Here's how the part is built. I have some questions about the finished solid (model axes, mm). A direction names the side the tool comes from. Give positions to 0.01 mm unless a question says otherwise; leave off trailing zeros. Write each loop counter-clockwise with the first axis right and the second up, starting at its lowest first coordinate (ties: lowest second). Pieces come first, ordered by that corner, then holes. Notation, with made-up numbers: (82.5, 34) -> (140.5, 34) arc R17 ccw to (140.5, 51) -> close; hole circle Ø9 at (1, 1). An arc over 180 degrees is marked (long way). Use CSV: the item, a comma, the result in double quotes. Start each with the question number.
(1) For pin 1 Ø3.5 at (x, y) = (-10, 0) entering from +Z; pin 2 Ø4 at (x, y) = (4, -3) entering from +Z, each with a flat end and sliding along its axis, tell me the tip position at first contact or that it passes through.
(2) Which directions (+Z, -Z, +X, -X, +Y, -Y) give clear straight access to the entire face, cutting with the end or side of a thin tool? Please do faces 1 (the cylindrical face through (-8.903, 0.345, 2.014)), 2 (the flat face through (-3.5, 0.1, 3)).
(3) Suppose I cut it at A-A on y = 0. List the corners of the cut face in (x, z) for me, plus the area to 3 significant figures.
(4) If we mould it in two halves opening along Y, with no side actions, what happens to faces 3 (the cylindrical face through (1.617, -0.67, 6.084)), 4 (the cylindrical face through (1.78, 7.18, 1.72)), 5 (the cylindrical face through (-1.78, -7.18, 1.72))? For each: pulls with the +Y half, pulls with the -Y half, needs draft (parallel to the pull), parting line crosses it, or undercut.
(5) Suppose I cut it at B-B on z = 10.25. List the corners of the cut face in (x, y) for me, plus the area to 3 significant figures.
(6) I need wall thicknesses on L1, parallel to Y at x = 10, z = 1.8; L2, parallel to Y at x = 0, z = 6.75; L3, parallel to Z at x = 3.5, y = -0.25. Which ranges of each line are inside material? Lowest first, please. Write a range as [from, to].
from build123d import *

# Parameters (mm, degrees)
F1_DEPTH      = 3
F2_T1_DEPTH   = 24.3364797517
F3_T1_DEPTH   = 14.1373136471
F4_R          = 3.25
F5_DEPTH      = 9
F6_R          = 1.75
F7_DEPTH      = 12.001
F8_SIZE       = 0.5
F4_R_2        = 1.15
F9_DEPTH      = 3.001
F10_SIZE      = 1
F11_T1_DEPTH  = 11.2158433332
F11_T3_DEPTH  = 11.2158433332
F11_T5_DEPTH  = 11.2158433332
F11_T7_DEPTH  = 11.2158433332
F11_T10_ANGLE = 127.4788590763
F11_T12_ANGLE = 42.4709850422
F11_T14_ANGLE = 42.4709850422
F11_T16_ANGLE = 42.4709850422
F11_T18_ANGLE = 42.4709850422
F11_T20_ANGLE = 127.4788590763


# Not quite as in the source:
# - a fillet or chamfer that OpenCascade refuses, or shapes differently, is made with other operations: its cross-section is extruded or revolved along the edge and cut away or added


with BuildPart() as f1:
    # F0 (on Top) → F1 (new body)
    with BuildSketch(Plane.XY):
        Polygon((-1.5, 7.5), (-17.5, 0), (-1.5, -7.5), (1.5, -7.5), (17.5, 0), (1.5, 7.5), align=None)
    extrude(amount=F1_DEPTH)

    # F2: fillet of radius 2 on 2 edges, made by hand

    # F2_s2 → F2_t1 (cut)
    with BuildSketch(Plane.XY.offset(-10.6682398759)):
        with BuildLine():
            ThreePointArc((-13.6363085399, 1.8115471368), (-14.7878407874, 0), (-13.6363085399, -1.8115471368))
            Line((-13.6363085399, -1.8115471368), (-13.7212248119, -1.9927018505))
            ThreePointArc((-13.7212248119, -1.9927018505), (-15.6529856552, -1.0867471903), (-17.584916272, -0.1811547137))
            Line((-17.584916272, -0.1811547137), (-17.584916272, 0.1811547137))
            ThreePointArc((-17.584916272, 0.1811547137), (-15.6529856552, 1.0867471903), (-13.7212248119, 1.9927018505))
            Line((-13.7212248119, 1.9927018505), (-13.6363085399, 1.8115471368))
        make_face()
        with BuildLine():
            ThreePointArc((13.6363085399, -1.8115471368), (14.7878407874, 0), (13.6363085399, 1.8115471368))
            Line((13.6363085399, 1.8115471368), (13.7212248119, 1.9927018505))
            ThreePointArc((13.7212248119, 1.9927018505), (15.6529856552, 1.0867471903), (17.584916272, 0.1811547137))
            Line((17.584916272, 0.1811547137), (17.584916272, -0.1811547137))
            ThreePointArc((17.584916272, -0.1811547137), (15.6529856552, -1.0867471903), (13.7212248119, -1.9927018505))
            Line((13.7212248119, -1.9927018505), (13.6363085399, -1.8115471368))
        make_face()
    extrude(amount=F2_T1_DEPTH, mode=Mode.SUBTRACT)

    # F3: fillet of radius 10 on 4 edges, made by hand

    # F3_s2 → F3_t1 (cut)
    with BuildSketch(Plane.XY.offset(-5.5686568236)):
        with BuildLine():
            ThreePointArc((-3.5168760329, 6.5545893596), (-1.4467160125, 7.2607861772), (0.7274627294, 7.5))
            Line((0.7274627294, 7.5), (-1.5, 7.5))
            Line((-1.5, 7.5), (-3.5168760329, 6.5545893596))
        make_face()
        with BuildLine():
            ThreePointArc((-0.7274627294, 7.5), (1.4467160125, 7.2607861772), (3.5168760329, 6.5545893596))
            Line((3.5168760329, 6.5545893596), (1.5, 7.5))
            Line((1.5, 7.5), (-0.7274627294, 7.5))
        make_face()
        with BuildLine():
            ThreePointArc((3.5168760329, -6.5545893596), (1.4467160125, -7.2607861772), (-0.7274627294, -7.5))
            Line((-0.7274627294, -7.5), (1.5, -7.5))
            Line((1.5, -7.5), (3.5168760329, -6.5545893596))
        make_face()
        with BuildLine():
            ThreePointArc((0.7274627294, -7.5), (-1.4467160125, -7.2607861772), (-3.5168760329, -6.5545893596))
            Line((-3.5168760329, -6.5545893596), (-1.5, -7.5))
            Line((-1.5, -7.5), (0.7274627294, -7.5))
        make_face()
    extrude(amount=F3_T1_DEPTH, mode=Mode.SUBTRACT)

    # F4 (on face) → F5 (join)
    with BuildSketch(Plane.XY.offset(3)):
        Circle(F4_R)
    extrude(amount=F5_DEPTH)

    # F6 (on face) → F7 (cut, through all)
    with BuildSketch(Plane.XY.offset(12)):
        Circle(F6_R)
    extrude(amount=-F7_DEPTH, mode=Mode.SUBTRACT)

    # F8
    f8_edges = [f1.edges().sort_by_distance(p)[0] for p in [
        (-3.25, 0, 12),
    ]]
    chamfer(f8_edges, length=F8_SIZE)

    # F4 (on face) → F9 (cut, through all)
    with BuildSketch(Plane.XY.offset(3)):
        with Locations((-10, 0)):
            Circle(F4_R_2)
        with Locations((10, 0)):
            Circle(F4_R_2)
    extrude(amount=-F9_DEPTH, mode=Mode.SUBTRACT)

    # F10
    f10_edges = [f1.edges().sort_by_distance(p)[0] for p in [
        (-11.15, 0, 0),
        (8.85, 0, 0),
    ]]
    chamfer(f10_edges, length=F10_SIZE)

    # F11: fillet of radius 0.5 on 10 edges, made by hand

    # F11_s2 → F11_t1 (cut)
    with BuildSketch(Plane(origin=(-10.5198395857, 4.9311748058, 0), x_dir=(0, 0, 1), z_dir=(0.905458936, -0.4244338762, 0))):
        with BuildLine():
            ThreePointArc((-0.0004, 6.9266271486), (0.1464466094, 7.2811462246), (0.5009656854, 7.427992834))
            Line((0.5009656854, 7.427992834), (0.5009656854, 7.4781294026))
            ThreePointArc((0.5009656854, 7.4781294026), (0.2504828427, 7.4777294026), (0, 7.4777294026))
            Line((0, 7.4777294026), (-0.0501365685, 7.427592834))
            ThreePointArc((-0.0501365685, 7.427592834), (-0.0501365685, 7.1771099913), (-0.0505365685, 6.9266271486))
            Line((-0.0505365685, 6.9266271486), (-0.0004, 6.9266271486))
        make_face()
    extrude(amount=F11_T1_DEPTH, mode=Mode.SUBTRACT)

    # F11_s4 → F11_t3 (cut)
    with BuildSketch(Plane(origin=(0.3643540153, 0.1707909447, 0), x_dir=(0, 0, 1), z_dir=(0.905458936, 0.4244338762, 0))):
        with BuildLine():
            ThreePointArc((-0.0004, 6.9266271486), (0.1464466094, 7.2811462246), (0.5009656854, 7.427992834))
            Line((0.5009656854, 7.427992834), (0.5009656854, 7.4781294026))
            ThreePointArc((0.5009656854, 7.4781294026), (0.2504828427, 7.4777294026), (0, 7.4777294026))
            Line((0, 7.4777294026), (-0.0501365685, 7.427592834))
            ThreePointArc((-0.0501365685, 7.427592834), (-0.0501365685, 7.1771099913), (-0.0505365685, 6.9266271486))
            Line((-0.0505365685, 6.9266271486), (-0.0004, 6.9266271486))
        make_face()
    extrude(amount=F11_T3_DEPTH, mode=Mode.SUBTRACT)

    # F11_s6 → F11_t5 (cut)
    with BuildSketch(Plane(origin=(10.5198395857, -4.9311748058, 0), x_dir=(0, 0, 1), z_dir=(-0.905458936, 0.4244338762, 0))):
        with BuildLine():
            ThreePointArc((-0.0004, 6.9266271486), (0.1464466094, 7.2811462246), (0.5009656854, 7.427992834))
            Line((0.5009656854, 7.427992834), (0.5009656854, 7.4781294026))
            ThreePointArc((0.5009656854, 7.4781294026), (0.2504828427, 7.4777294026), (0, 7.4777294026))
            Line((0, 7.4777294026), (-0.0501365685, 7.427592834))
            ThreePointArc((-0.0501365685, 7.427592834), (-0.0501365685, 7.1771099913), (-0.0505365685, 6.9266271486))
            Line((-0.0505365685, 6.9266271486), (-0.0004, 6.9266271486))
        make_face()
    extrude(amount=F11_T5_DEPTH, mode=Mode.SUBTRACT)

    # F11_s8 → F11_t7 (cut)
    with BuildSketch(Plane(origin=(-0.3643540153, -0.1707909447, 0), x_dir=(0, 0, 1), z_dir=(-0.905458936, -0.4244338762, 0))):
        with BuildLine():
            ThreePointArc((-0.0004, 6.9266271486), (0.1464466094, 7.2811462246), (0.5009656854, 7.427992834))
            Line((0.5009656854, 7.427992834), (0.5009656854, 7.4781294026))
            ThreePointArc((0.5009656854, 7.4781294026), (0.2504828427, 7.4777294026), (0, 7.4777294026))
            Line((0, 7.4777294026), (-0.0501365685, 7.427592834))
            ThreePointArc((-0.0501365685, 7.427592834), (-0.0501365685, 7.1771099913), (-0.0505365685, 6.9266271486))
            Line((-0.0505365685, 6.9266271486), (-0.0004, 6.9266271486))
        make_face()
    extrude(amount=F11_T7_DEPTH, mode=Mode.SUBTRACT)

    # F11_s9 → F11_t10 (revolve, cut)
    with BuildSketch(Plane(origin=(10.283861632, -5.0737982035, 0), x_dir=(0, 0, 1), z_dir=(-0.8967911287, 0.4424541462, 0))):
        with BuildLine():
            ThreePointArc((-0.0004, 7.157454968), (0.1464466094, 7.511974044), (0.5009656854, 7.6588206534))
            Line((0.5009656854, 7.6588206534), (0.5009656854, 7.708957222))
            ThreePointArc((0.5009656854, 7.708957222), (0.2504828427, 7.708557222), (0, 7.708557222))
            Line((0, 7.708557222), (-0.0501365685, 7.6584206534))
            ThreePointArc((-0.0501365685, 7.6584206534), (-0.0501365685, 7.4079378107), (-0.0505365685, 7.157454968))
            Line((-0.0505365685, 7.157454968), (-0.0004, 7.157454968))
        make_face()
    revolve(axis=Axis((12.7871458195, 0, 0), (0, 0, -1)), revolution_arc=F11_T10_ANGLE, mode=Mode.SUBTRACT)

    # F11_s11 → F11_t12 (revolve, cut)
    with BuildSketch(Plane(origin=(-1.3745464916, -0.429601751, 0), x_dir=(0, 0, 1), z_dir=(-0.9544689122, -0.2983104016, 0))):
        with BuildLine():
            ThreePointArc((-0.0004, 7.3298717335), (0.1464466094, 7.6843908095), (0.5009656854, 7.8312374189))
            Line((0.5009656854, 7.8312374189), (0.5009656854, 7.8813739874))
            ThreePointArc((0.5009656854, 7.8813739874), (0.2504828427, 7.8809739874), (0, 7.8809739874))
            Line((0, 7.8809739874), (-0.0501365685, 7.8308374189))
            ThreePointArc((-0.0501365685, 7.8308374189), (-0.0501365685, 7.5803545762), (-0.0505365685, 7.3298717335))
            Line((-0.0505365685, 7.3298717335), (-0.0004, 7.3298717335))
        make_face()
    revolve(axis=Axis((-0.72746273, -2.5000000027, 0), (0, 0, -1)), revolution_arc=F11_T12_ANGLE, mode=Mode.SUBTRACT)

    # F11_s13 → F11_t14 (revolve, cut)
    with BuildSketch(Plane(origin=(-0.3643540157, -0.1707909448, 0), x_dir=(0, 0, 1), z_dir=(-0.905458936, -0.4244338762, 0))):
        with BuildLine():
            ThreePointArc((-0.0004, 6.9266271486), (0.1464466094, 7.2811462246), (0.5009656854, 7.427992834))
            Line((0.5009656854, 7.427992834), (0.5009656854, 7.4781294026))
            ThreePointArc((0.5009656854, 7.4781294026), (0.2504828427, 7.4777294026), (0, 7.4777294026))
            Line((0, 7.4777294026), (-0.0501365685, 7.427592834))
            ThreePointArc((-0.0501365685, 7.427592834), (-0.0501365685, 7.1771099913), (-0.0505365685, 6.9266271486))
            Line((-0.0505365685, 6.9266271486), (-0.0004, 6.9266271486))
        make_face()
    revolve(axis=Axis((0.72746273, -2.5000000027, 0), (0, 0, -1)), revolution_arc=F11_T14_ANGLE, mode=Mode.SUBTRACT)

    # F11_s15 → F11_t16 (revolve, cut)
    with BuildSketch(Plane(origin=(0.3643540157, 0.1707909448, 0), x_dir=(0, 0, 1), z_dir=(0.905458936, 0.4244338762, 0))):
        with BuildLine():
            ThreePointArc((-0.0004, 6.9266271486), (0.1464466094, 7.2811462246), (0.5009656854, 7.427992834))
            Line((0.5009656854, 7.427992834), (0.5009656854, 7.4781294026))
            ThreePointArc((0.5009656854, 7.4781294026), (0.2504828427, 7.4777294026), (0, 7.4777294026))
            Line((0, 7.4777294026), (-0.0501365685, 7.427592834))
            ThreePointArc((-0.0501365685, 7.427592834), (-0.0501365685, 7.1771099913), (-0.0505365685, 6.9266271486))
            Line((-0.0505365685, 6.9266271486), (-0.0004, 6.9266271486))
        make_face()
    revolve(axis=Axis((-0.72746273, 2.5000000027, 0), (0, 0, -1)), revolution_arc=F11_T16_ANGLE, mode=Mode.SUBTRACT)

    # F11_s17 → F11_t18 (revolve, cut)
    with BuildSketch(Plane(origin=(1.3745464916, 0.429601751, 0), x_dir=(0, 0, 1), z_dir=(0.9544689122, 0.2983104016, 0))):
        with BuildLine():
            ThreePointArc((-0.0004, 7.3298717335), (0.1464466094, 7.6843908095), (0.5009656854, 7.8312374189))
            Line((0.5009656854, 7.8312374189), (0.5009656854, 7.8813739874))
            ThreePointArc((0.5009656854, 7.8813739874), (0.2504828427, 7.8809739874), (0, 7.8809739874))
            Line((0, 7.8809739874), (-0.0501365685, 7.8308374189))
            ThreePointArc((-0.0501365685, 7.8308374189), (-0.0501365685, 7.5803545762), (-0.0505365685, 7.3298717335))
            Line((-0.0505365685, 7.3298717335), (-0.0004, 7.3298717335))
        make_face()
    revolve(axis=Axis((0.72746273, 2.5000000027, 0), (0, 0, -1)), revolution_arc=F11_T18_ANGLE, mode=Mode.SUBTRACT)

    # F11_s19 → F11_t20 (revolve, cut)
    with BuildSketch(Plane(origin=(-10.283861632, 5.0737982035, 0), x_dir=(0, 0, 1), z_dir=(0.8967911287, -0.4424541462, 0))):
        with BuildLine():
            ThreePointArc((-0.0004, 7.157454968), (0.1464466094, 7.511974044), (0.5009656854, 7.6588206534))
            Line((0.5009656854, 7.6588206534), (0.5009656854, 7.708957222))
            ThreePointArc((0.5009656854, 7.708957222), (0.2504828427, 7.708557222), (0, 7.708557222))
            Line((0, 7.708557222), (-0.0501365685, 7.6584206534))
            ThreePointArc((-0.0501365685, 7.6584206534), (-0.0501365685, 7.4079378107), (-0.0505365685, 7.157454968))
            Line((-0.0505365685, 7.157454968), (-0.0004, 7.157454968))
        make_face()
    revolve(axis=Axis((-12.7871458195, 0, 0), (0, 0, -1)), revolution_arc=F11_T20_ANGLE, mode=Mode.SUBTRACT)


solid = f1.part
Geometry says:
1,pin 1,"z = 3"
1,pin 2,"z = 11.75"
2,face 1,"+Z, -Z"
2,face 2,"+Z"
3,outline,"(-14.79, 0.48) arc R0.5 ccw to (-14.31, 0) -> (-12.15, 0) -> (-11.15, 1) -> (-11.15, 3) -> (-14.79, 3) -> close; (-8.85, 1) -> (-7.85, 0) -> (-1.75, 0) -> (-1.75, 12) -> (-2.75, 12) -> (-3.25, 11.5) -> (-3.25, 3) -> (-8.85, 3) -> close; (1.75, 0) -> (7.85, 0) -> (8.85, 1) -> (8.85, 3) -> (3.25, 3) -> (3.25, 11.5) -> (2.75, 12) -> (1.75, 12) -> close; (11.15, 1) -> (12.15, 0) -> (14.31, 0) arc R0.5 ccw to (14.79, 0.48) -> (14.79, 3) -> (11.15, 3) -> close"
3,area,"89.1 mm²"
4,face 3,"undercut"
4,face 4,"pulls with the +Y half"
4,face 5,"pulls with the -Y half"
5,outline,"circle Ø6.5 at (0, 0); hole circle Ø3.5 at (0, 0)"
5,area,"23.6 mm²"
6,L1,"[-3.52, -1.15], [1.15, 3.52]"
6,L2,"[-3.25, -1.75], [1.75, 3.25]"
6,L3,"[0, 3]"
